Could you check a few things on this model? Use its own coordinates, in mm. A direction names the side the tool comes from. Give positions to 0.01 mm unless a question says otherwise; leave off trailing zeros. Loops run counter-clockwise (first coordinate to the right, second up) from the corner with the lowest first, then second, coordinate; pieces in that order, holes last. Notation, with made-up numbers: M -6.5,40 L 7.5,40 A18 cw 7.5,58 Z; hole C 50.25,72.25 d1. An arc over 180 degrees is marked long. Answer in a Markdown table with one row per item. Add a question column.
```python
from build123d import *

# Parameters (mm, degrees)
F0_W     = 160.1980030537
F0_H     = 133.0576241016
F1_DEPTH = 133.096
F2_R     = 50.8
F3_T     = -2.54


# Not quite as in the source:
# - a shell that OpenCascade refuses in one call is made with other operations: the cavity is built on its own and cut out


with BuildPart() as f1:
    # F0 (on Front) → F1 (new body)
    with BuildSketch(Plane.XZ):
        with Locations((-80.0990015268, 66.5288120508)):
            Rectangle(F0_W, F0_H)
    extrude(amount=F1_DEPTH)

    # F2
    f2_edges = [f1.edges().sort_by_distance(p)[0] for p in [
        (-80.099002, -133.096, 133.057624),
    ]]
    fillet(f2_edges, radius=F2_R)

    # F3: a shell. OpenCascade refuses it in one call, so the cavity is built on its own and cut out:
    # the body offset inwards by the wall thickness, plus a prism from it out through each open face.
    f3_core = offset(f1.part, amount=F3_T, mode=Mode.PRIVATE)
    f3_exits = [f3_core.faces().sort_by_distance(p)[0] for p in [
        (-80.099002, -42.418, 130.517624),
    ]]
    add(f3_core, mode=Mode.SUBTRACT)
    extrude(f3_exits, amount=-F3_T, mode=Mode.SUBTRACT)


solid = f1.part
```
Item 1: If we mould it in two halves opening along Y, with no side actions, what happens to faces 4 (the face through (-81, -133.096, 42)), 5 (the face through (-81, -66, 0)), 6 (the face through (-81, -66, 2.54)), 7 (the face through (-2.54, -66, 67))? For each: +Y half, -Y half, draft (parallel to the pull), parting line (faces both ways), or undercut.
Item 2: Suppose I cut it at B-B (x = -106). List the corners of the cut face in (y, z) for me, then the cut area to 3 significant figures.
Item 3: I need wall thicknesses on L1, parallel to X at y = -111, z = 7; L2, parallel to Y at x = -64.5, z = 70.5; L3, parallel to Z at x = -68, y = -111.5. Which ranges of each line are inside material? Lowest first, please.
Item 4: Suppose I cut it at D-D (y = -111). List the corners of the cut face in (x, z) for me, then the cut area to 3 significant figures.
Item 5: For P1, Ø10, axis at x = -129.5, y = -48.5, coming from the +Z side; P2, Ø10, axis at x = -18, z = 107.5, coming from the -Y side, each with a flat end and sliding along its axis, tell me the tip position at first contact or that it passes through.
Item 6: Suppose I cut it at C-C (y = -78.5). List the corners of the cut face in (x, z) for me.
Item 7: Suppose I cut it at A-A (z = 70). List the corners of the cut face in (x, y) for me.
Item 8: For faces 1 (the face through (-80, -1, 133.058)), 2 (the face through (-79, -2.54, 67)), 3 (the face through (-79, -116, 116.8)), which set-ups out of +Z, -Z, +X, -X, +Y, -Y let a thin tool reach every point of the face, with its end or its side?
Values found:
| question | item | result |
|---|---|---|
| 1 | face 4 | -Y half |
| 1 | face 5 | draft |
| 1 | face 6 | undercut |
| 1 | face 7 | undercut |
| 2 | outline | M -133.1,0 L 0,0 L 0,133.06 L -2.54,133.06 L -2.54,2.54 L -130.56,2.54 L -130.56,82.26 A48.26 cw -82.3,130.52 L -82.3,133.06 A50.8 ccw -133.1,82.26 Z |
| 2 | area | 1,070 mm² |
| 3 | L1 | -160.2 to -157.66, -2.54 to 0 |
| 3 | L2 | -133.1 to -130.56, -2.54 to 0 |
| 3 | L3 | 0 to 2.54, 120.68 to 123.82 |
| 4 | outline | M -160.2,0 L 0,0 L 0,124.17 L -160.2,124.17 Z; hole M -157.66,2.54 L -2.54,2.54 L -2.54,121.05 L -157.66,121.05 Z |
| 4 | area | 1,510 mm² |
| 5 | P1 | z = 2.54 |
| 5 | P2 | y = -128.89 |
| 6 | outline | M -160.2,0 L 0,0 L 0,133.06 L -2.54,133.06 L -2.54,2.54 L -157.66,2.54 L -157.66,133.06 L -160.2,133.06 Z |
| 7 | outline | M -160.2,-133.1 L 0,-133.1 L 0,0 L -160.2,0 Z; hole M -157.66,-130.56 L -2.54,-130.56 L -2.54,-2.54 L -157.66,-2.54 Z |
| 8 | face 1 | +Z, +X, -X, +Y, -Y |
| 8 | face 2 | +Z |
| 8 | face 3 | none |
